Read the model definition and answer for the solid it produces. Units are mm, in the model's axes. Face numbers are marked on the shaded views. A direction names the side the tool comes from. Coordinates: 2 decimals unless noted, no trailing zeros. Loops run counter-clockwise (first coordinate to the right, second up) from the corner with the lowest first, then second, coordinate; pieces in that order, holes last. Notation, with made-up numbers: (-35, -36) - (0, -36) arc R26 ccw to (0, -20) - close; hole circle Ø6 at (89.5, -31). An arc over 180 degrees is marked (long way). One line per question, with ' | ' between items. Start each with the question number.
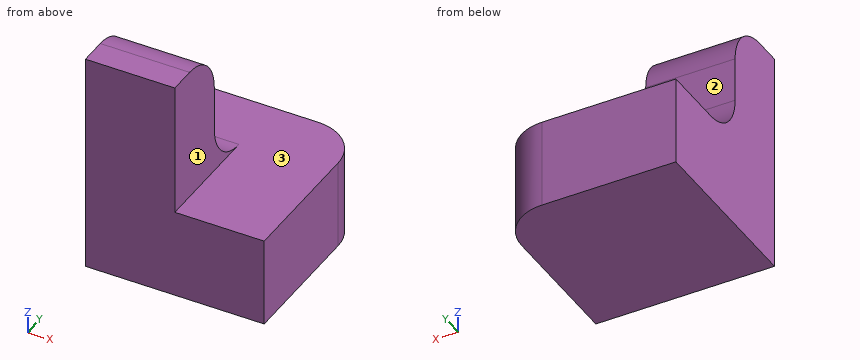
```python
from build123d import *

# Parameters (mm, degrees)
SKETCH1_W           = 20
SKETCH1_H           = 16
BOSS_EXTRUDE1_DEPTH = 30
SKETCH2_W           = 40
SKETCH2_H           = 40
BOSS_EXTRUDE2_DEPTH = 20
FILLET1_R           = 10


with BuildPart() as part:
    # Sketch1 → Boss-Extrude1 (new body)
    with BuildSketch(Plane.XY):
        with Locations((-20, -8)):
            Rectangle(SKETCH1_W, SKETCH1_H)
    extrude(amount=BOSS_EXTRUDE1_DEPTH)

    # Sketch2 → Boss-Extrude2 (add)
    with BuildSketch(Plane.XY):
        with Locations((-10, 4)):
            Rectangle(SKETCH2_W, SKETCH2_H)
    extrude(amount=-BOSS_EXTRUDE2_DEPTH)

    # Fillet1
    fillet1_edges = [part.edges().sort_by_distance(p)[0] for p in [
        (10, 24, -10),
        (-20, 0, 30),
        (-20, 0, 0),
    ]]
    fillet(fillet1_edges, radius=FILLET1_R)


solid = part.part
```
1) The part is cut by section D-D on y = 4. Write down the section's boundary in (x, z), and give its area (3 significant figures).
2) Which of the six approach directions +Z, -Z, +X, -X, +Y, -Y give full straight-line access (tool end or side, diameter ignored) to the marked faces 1, 2 and 3?
3) The part is cut by section A-A on x = -19. Write down the section's boundary in (y, z).
4) The part is cut by section B-B on y = -12.5. Write down the section's boundary in (x, z).
5) Given pin 1 Ø6 at (y, z) = (-8.5, 5) entering from +X; pin 2 Ø5 at (x, y) = (-23.5, 4) entering from +Z; pin 3 Ø8 at (x, z) = (-20, 13) entering from +Y, each flat-ended and moving along its own axis, determine where each tip first touches the part or whether it passes through.
6) Find the intervals of material crossed by line 1 along X through (y, z) = (-7.5, 0.5); line 2 along Z through (x, y) = (-3.5, 11); line 3 along Z through (x, y) = (-27.5, -9.5), in increasing order. Write a range as from..to.
7) The part is cut by section C-C on z = 26. Write down the section's boundary in (x, y).
Answer below:
1) outline: (-30, -20) - (10, -20) - (10, 0) - (-10, 0) - (-10, 2) - (-30, 2) - close | area: 840 mm2
2) face 1: +Z, +X, +Y, -Y | face 2: +Z, +X, -X, +Y | face 3: +Z, +X, +Y
3) outline: (-16, -20) - (24, -20) - (24, 0) - (10, 0) arc R10 cw to (0, 10) - (0, 20) arc R10 ccw to (-10, 30) - (-16, 30) - close
4) outline: (-30, -20) - (10, -20) - (10, 0) - (-10, 0) - (-10, 30) - (-30, 30) - close
5) pin 1: x = -10 | pin 2: z = 4.73 | pin 3: y = 0.05
6) line 1: -30..-10 | line 2: -20..0 | line 3: -20..29.99
7) outline: (-30, -16) - (-10, -16) - (-10, -2) - (-30, -2) - close
